Input: part model. Units: mm. Frame: model coordinates. A direction names the side the tool comes from. Coordinates: 2 decimals unless noted, no trailing zeros. Write each loop counter-clockwise with the first axis right and the second up, starting at its lowest first coordinate (ties: lowest second). Pieces come first, ordered by that corner, then holes. Notation, with made-up numbers: (-24, -27) - (-18, -27) arc R19 cw to (-18, -14) - close; hole circle Ø1 at (21.25, -5). An arc over 180 degrees is marked (long way). Use CSV: the item, a comma, the result in double quotes.
```python
from build123d import *

# Parameters (mm, degrees)
BOSS_EXTRUDE1_DEPTH  = 83.0326
SKETCH2_W            = 61.8998
SKETCH2_H            = 21.463
BOSS_EXTRUDE2_DEPTH  = 3.175
SKETCH3_W            = 25.4
SKETCH3_H            = 5.08
CUT_EXTRUDE1_DEPTH   = 107.886039958
FILLET1_R            = 0.762
FILLET2_R            = 0.762
FILLET3_R            = 0.762
SKETCH5_W            = 16.529901782
SKETCH5_H            = 9.525
CUT_EXTRUDE2_DEPTH   = 90.51870739
SKETCH41_W           = 86.2076
SKETCH41_H           = 30.988
BOSS_EXTRUDE10_DEPTH = 1.5875
SKETCH42_W           = 86.2076
SKETCH42_H           = 1.5875
BOSS_EXTRUDE11_DEPTH = 25.4
SKETCH47_W           = 86.2076
SKETCH47_H           = 1.5875
BOSS_EXTRUDE13_DEPTH = 25.4
SKETCH48_W           = 86.2076
SKETCH48_H           = 30.988
BOSS_EXTRUDE14_DEPTH = 1.5875
SKETCH49_W           = 1.5875
SKETCH49_H           = 16.764
CUT_EXTRUDE5_DEPTH   = 35.56
SKETCH50_W           = 6.35
SKETCH50_H           = 1.5875
BOSS_EXTRUDE15_DEPTH = 9.2075
SKETCH52_W           = 6.35
SKETCH52_H           = 30.988
BOSS_EXTRUDE17_DEPTH = 1.5875
SKETCH53_W           = 25.4
SKETCH53_H           = 61.8998
CUT_EXTRUDE6_DEPTH   = 3.175


with BuildPart() as part:
    # Sketch1 → Boss-Extrude1 (new body)
    with BuildSketch(Plane(origin=(0, 0, 0), x_dir=(0, 0, -1), z_dir=(1, 0, 0))):
        Polygon((-27.7749, 9.525), (-24.0411, 9.525), (-24.0411, 12.7), (-30.9499, 12.7), (-30.9499, -3.175), (-30.9499, -8.763), (30.9499, -8.763), (30.9499, -3.175), (30.9499, 12.7), (24.0411, 12.7), (24.0411, 9.525), (27.7749, 9.525), (27.7749, 0), (-27.7749, 0), align=None)
    extrude(amount=BOSS_EXTRUDE1_DEPTH)

    # Sketch2 → Boss-Extrude2 (add)
    with BuildSketch(Plane(origin=(83.0326, 0, 0), x_dir=(0, 0, -1), z_dir=(1, 0, 0))):
        with Locations((0, 1.9685)):
            Rectangle(SKETCH2_W, SKETCH2_H)
    extrude(amount=BOSS_EXTRUDE2_DEPTH)

    # Sketch3 → Cut-Extrude1 (cut, through all)
    with BuildSketch(Plane.XY.offset(30.9499)):
        with Locations((24.0538, -4.815937668)):
            Rectangle(SKETCH3_W, SKETCH3_H)
        with Locations((62.1538, -4.815937668)):
            Rectangle(SKETCH3_W, SKETCH3_H)
    extrude(amount=-CUT_EXTRUDE1_DEPTH, mode=Mode.SUBTRACT)

    # Fillet1
    fillet1_edges = [part.edges().sort_by_distance(p)[0] for p in [
        (24.0538, -7.355937668, -30.9499),
        (24.0538, -7.355937668, 30.9499),
        (62.1538, -7.355937668, -30.9499),
        (62.1538, -7.355937668, 30.9499),
    ]]
    fillet(fillet1_edges, radius=FILLET1_R)

    # Fillet2
    fillet2_edges = [part.edges().sort_by_distance(p)[0] for p in [
        (11.3538, -5.196937668, -30.9499),
        (24.0538, -2.275937668, -30.9499),
        (36.7538, -5.196937668, -30.9499),
        (49.4538, -5.196937668, -30.9499),
        (62.1538, -2.275937668, -30.9499),
        (74.8538, -5.196937668, -30.9499),
    ]]
    fillet(fillet2_edges, radius=FILLET2_R)

    # Fillet3
    fillet3_edges = [part.edges().sort_by_distance(p)[0] for p in [
        (74.8538, -5.196937668, 30.9499),
        (62.1538, -2.275937668, 30.9499),
        (49.4538, -5.196937668, 30.9499),
        (11.3538, -5.196937668, 30.9499),
        (24.0538, -2.275937668, 30.9499),
        (36.7538, -5.196937668, 30.9499),
    ]]
    fillet(fillet3_edges, radius=FILLET3_R)

    # Sketch5 → Cut-Extrude2 (cut, through all)
    with BuildSketch(Plane.ZY.offset(-83.0326)):
        with Locations((0, 4.7625)):
            Rectangle(SKETCH5_W, SKETCH5_H)
    extrude(amount=-CUT_EXTRUDE2_DEPTH, mode=Mode.SUBTRACT)

    # Sketch41 → Boss-Extrude10 (add)
    with BuildSketch(Plane.XY.offset(30.9499)):
        with Locations((43.1038, 15.494)):
            Rectangle(SKETCH41_W, SKETCH41_H)
    extrude(amount=BOSS_EXTRUDE10_DEPTH)

    # Sketch42 → Boss-Extrude11 (add)
    with BuildSketch(Plane.XY.offset(32.5374)):
        with Locations((43.1038, 0.79375)):
            Rectangle(SKETCH42_W, SKETCH42_H)
    extrude(amount=BOSS_EXTRUDE11_DEPTH)

    # Sketch47 → Boss-Extrude13 (add)
    with BuildSketch(Plane.XY.offset(32.5374)):
        with Locations((43.1038, 30.19425)):
            Rectangle(SKETCH47_W, SKETCH47_H)
    extrude(amount=BOSS_EXTRUDE13_DEPTH)

    # Sketch48 → Boss-Extrude14 (add)
    with BuildSketch(Plane.XY.offset(57.9374)):
        with Locations((43.1038, 15.494)):
            Rectangle(SKETCH48_W, SKETCH48_H)
    extrude(amount=BOSS_EXTRUDE14_DEPTH)

    # Sketch49 → Cut-Extrude5 (cut)
    with BuildSketch(Plane.ZY):
        with Locations((58.73115, 15.494)):
            Rectangle(SKETCH49_W, SKETCH49_H)
    extrude(amount=-CUT_EXTRUDE5_DEPTH, mode=Mode.SUBTRACT)

    # Sketch50 → Boss-Extrude15 (add)
    with BuildSketch(Plane(origin=(86.2076, 0, 0), x_dir=(0, 0, -1), z_dir=(1, 0, 0))):
        with Locations((-45.2374, 30.19425)):
            Rectangle(SKETCH50_W, SKETCH50_H)
        with Locations((-45.2374, 0.79375)):
            Rectangle(SKETCH50_W, SKETCH50_H)
    extrude(amount=BOSS_EXTRUDE15_DEPTH)

    # Sketch52 → Boss-Extrude17 (add)
    with BuildSketch(Plane(origin=(95.4151, 0, 0), x_dir=(0, 0, -1), z_dir=(1, 0, 0))):
        with Locations((-45.2374, 15.494)):
            Rectangle(SKETCH52_W, SKETCH52_H)
    extrude(amount=BOSS_EXTRUDE17_DEPTH)

    # Sketch53 → Cut-Extrude6 (cut)
    with BuildSketch(Plane(origin=(0, 12.7, 0), x_dir=(1, 0, 0), z_dir=(0, 1, 0))):
        with Locations((12.7, 0)):
            Rectangle(SKETCH53_W, SKETCH53_H)
    extrude(amount=-CUT_EXTRUDE6_DEPTH, mode=Mode.SUBTRACT)


solid = part.part
```
(1) Cut plane C-C on z = 35. Return loops of the section in (x, y), and give its area (3 significant figures).
Check values:
outline,"(0, 0) - (86.21, 0) - (86.21, 1.59) - (0, 1.59) - close; (0, 29.4) - (86.21, 29.4) - (86.21, 30.99) - (0, 30.99) - close"
area,"274 mm^2"
(2) Cut plane B-B on y = -5.5. Return loops of the section in (x, z), and give its area (3 significant figures).
Check values:
outline,"(0, -30.95) - (10.59, -30.95) arc R0.76 ccw to (11.35, -30.19) - (11.35, 30.19) arc R0.76 ccw to (10.59, 30.95) - (0, 30.95) - close; (36.75, -30.19) arc R0.76 ccw to (37.52, -30.95) - (48.69, -30.95) arc R0.76 ccw to (49.45, -30.19) - (49.45, 30.19) arc R0.76 ccw to (48.69, 30.95) - (37.52, 30.95) arc R0.76 ccw to (36.75, 30.19) - close; (74.85, -30.19) arc R0.76 ccw to (75.62, -30.95) - (86.21, -30.95) - (86.21, 30.95) - (75.62, 30.95) arc R0.76 ccw to (74.85, 30.19) - close"
area,"2,190 mm^2"
(3) Reachability of faces 4 (the flat face through (85, 5, 8.265)), 5 (the flat face through (43, -4, 30.95)), 6 (the flat face through (41, 5, -27.775)), 7 (the flat face through (49.454, -5, 0)) from +Z, -Z, +X, -X, +Y, -Y: full face, straight path, thin tool, end or side. Return the list, or none.
Check values:
face 4,"+X, -X"
face 5,"+Z, +X, -X, -Y"
face 6,"-X"
face 7,"+Z, -Z"
(4) Cut plane A-A on x = 89.5. Return loops of the section in (y, z).
Check values:
outline,"(0, 42.06) - (1.59, 42.06) - (1.59, 48.41) - (0, 48.41) - close; (29.4, 42.06) - (30.99, 42.06) - (30.99, 48.41) - (29.4, 48.41) - close"
(5) Draft query along X for faces 1 (the flat face through (11.354, -5, 0)), 2 (the flat face through (54, 11, -24.041)), 3 (the flat face through (25.4, 11, -27)). Return one class per face: pulls with the +X half, pulls with the -X half, needs draft (parallel to the pull), parting line crosses it, or undercut.
Check values:
face 1,"undercut"
face 2,"needs draft"
face 3,"pulls with the -X half"
(6) Pin query (flat end, axial travel): pin 1 Ø3.5 at (y, z) = (10.5, 27) entering from -X; pin 2 Ø1 at (y, z) = (11, -5) entering from -X; pin 3 Ø20.5 at (x, z) = (29, -1.5) entering from +Y; pin 4 Ø6 at (x, y) = (79.5, 26.5) entering from -Z. Return the tip coordinate at first contact, or that it passes through.
Check values:
pin 1,"x = 0"
pin 2,"x = 83.03"
pin 3,"y = 0"
pin 4,"z = 30.95"
(7) Ray query, probe 1 along X at (y, z) = (-6, -22); probe 2 along Z at (x, y) = (63, 3); probe 3 along Y at (x, z) = (27, -5). Return the intervals inside material, ascending. Write a range as from..to.
Check values:
probe 1,"0..11.35, 36.75..49.45, 74.85..86.21"
probe 2,"-30.95..-27.77, 27.77..32.54, 57.94..59.52"
probe 3,"-8.76..-7.36, -2.28..0"
(8) Cut plane D-D on x = 65. Return loops of the section in (y, z) (1 decimal).
Check values:
outline,"(-8.8, -30.9) - (-8.1, -30.9) arc R0.8 ccw to (-7.4, -30.2) - (-7.4, 30.2) arc R0.8 ccw to (-8.1, 30.9) - (-8.8, 30.9) - close; (-2.3, -30.2) arc R0.8 ccw to (-1.5, -30.9) - (12.7, -30.9) - (12.7, -24) - (9.5, -24) - (9.5, -27.8) - (0, -27.8) - (0, 27.8) - (9.5, 27.8) - (9.5, 24) - (12.7, 24) - (12.7, 30.9) - (31, 30.9) - (31, 59.5) - (0, 59.5) - (0, 30.9) - (-1.5, 30.9) arc R0.8 ccw to (-2.3, 30.2) - close; hole (1.6, 32.5) - (29.4, 32.5) - (29.4, 57.9) - (1.6, 57.9) - close"
